Input: part model. Units: mm. Frame: model coordinates. A direction names the side the tool comes from. Round coordinates to 2 decimals unless told otherwise and drop trailing zeros. Loops run counter-clockwise (first coordinate to the right, second up) from the corner with the lowest first, then second, coordinate; pieces in that order, holes last. Notation, with made-up numbers: M 53.25,-2 L 96.25,-2 A10 cw 96.25,12 Z; hole C 60,81 d4. An arc over 180 degrees is marked long. Return JSON: item names as keys, results as strings. Group by question number.
1) Mould query, pull axis Z, two halves, no side actions, for faces 1 (the face through (-166, 3, -15)), 2 (the face through (-378.65, 1.48, 8.9)), 3 (the face through (-4.88, 1.48, -1.08)). Classes: +Z half, -Z half, draft (parallel to the pull), parting line (faces both ways), or undercut.
2) Section C-C (x = -40). Output: boundary loops of the cut face in (y, z).
3) Contact query for flat-ended pins moving along their axis: P1, Ø0.9, axis at x = 20.5, y = 1.5, coming from the -Z side; P2, Ø6, axis at x = 0, z = 0, coming from the -Y side. Output: stop coordinate, or through.
4) Section B-B (x = -227). Output: boundary loops of the cut face in (y, z), plus the area to 3 significant figures.
5) Material intervals for line 1 (Z direction, x = 20, y = 0.15); line 2 (Z direction, x = -91, y = 0.2), sorted ascending. Write a range as from..to.
6) Access query for faces 4 (the face through (55, 1, 0)), 5 (the face through (-322.106, 1.479, 17.412)). Directions: +Z, -Z, +X, -X, +Y, -Y. A direction counts if a zero-diameter tool reaches every point of the face in a straight line with its end or side. Return the directions, or none.
7) Section A-A (y = 0.75). Count the separate pieces of the cut face and the enclosed holes in it, plus the area to 3 significant figures.
from build123d import *

# Parameters (mm, degrees)
SKETCH1_R           = 5
SKETCH1_R_2         = 2
BOSS_EXTRUDE1_DEPTH = 3
FILLET1_R           = 100


with BuildPart() as part:
    # Sketch1 → Boss-Extrude1 (new body)
    with BuildSketch(Plane(origin=(0, 0, 0), x_dir=(1, 0, 0), z_dir=(0, 1, 0))):
        with BuildLine():
            Line((0, 15), (-139.784941349, 43.225909045))
            Line((-139.784941349, 43.225909045), (-351.875415017, 29.941322925))
            ThreePointArc((-351.875415017, 29.941322925), (-378.412739548, -9.628926804), (-333.285739517, -24.912516864))
            Line((-333.285739517, -24.912516864), (-287.823465989, 5.588948968))
            Line((-287.823465989, 5.588948968), (-138.053278996, 13.889014505))
            Line((-138.053278996, 13.889014505), (-5.919683, -13.782501703))
            Line((-5.919683, -13.782501703), (0, -15))
            Line((0, -15), (40, -15))
            ThreePointArc((40, -15), (55, 0), (40, 15))
            Line((40, 15), (0, 15))
        make_face()
        with Locations(Location((0, 0, 0), (0, 0, 270))):
            Circle(SKETCH1_R, mode=Mode.SUBTRACT)
        with Locations(Location((40, 0, 0), (0, 0, 270))):
            Circle(SKETCH1_R_2, mode=Mode.SUBTRACT)
    extrude(amount=BOSS_EXTRUDE1_DEPTH)

    # Fillet1
    fillet1_edges = [part.edges().sort_by_distance(p)[0] for p in [
        (0, 1.5, -15),
        (-139.784941349, 1.5, -43.225909045),
        (-138.053278996, 1.5, -13.889014505),
        (-287.823465989, 1.5, -5.588948968),
        (0, 1.5, 15),
    ]]
    fillet(fillet1_edges, radius=FILLET1_R)


solid = part.part
Returned:
{
 "1": {"face 1": "draft", "face 2": "parting line", "face 3": "undercut"},
 "2": {"outline": "M 0,-23.08 L 3,-23.08 L 3,6.65 L 0,6.65 Z"},
 "3": {"P1": "stops at z = -15", "P2": "passes through"},
 "4": {"outline": "M 0,-37.76 L 3,-37.76 L 3,-8.96 L 0,-8.96 Z", "area": "86.4 mm^2"},
 "5": {"line 1": "z = -15..15", "line 2": "z = -33.38..-4.04"},
 "6": {"face 4": "+X, +Y, -Y", "face 5": "+Z, +Y, -Y"},
 "7": {"separate pieces": "1", "enclosed holes": "2", "area": "14,200 mm^2"}
}
